from build123d import *

# Parameters (mm, degrees)
SKETCH1_W           = 49
SKETCH1_H           = 49
SKETCH1_W_2         = 4
SKETCH1_H_2         = 5
SKETCH1_W_3         = 3
BOSS_EXTRUDE1_DEPTH = 3


with BuildPart() as part:
    # Sketch1 → Boss-Extrude1 (new body)
    with BuildSketch(Plane(origin=(0, 0, 0), x_dir=(1, 0, 0), z_dir=(0, 1, 0))):
        Rectangle(SKETCH1_W, SKETCH1_H)
        with Locations((26.5, 0)):
            Rectangle(SKETCH1_W_2, SKETCH1_H_2)
        Polygon((-27.5, 27.5), (-27.5, 24.5), (-27.5, -24.5), (-27.5, -27.5), (-30.5, -27.5), (-30.5, 27.5), align=None)
        with Locations((-26, 0)):
            Rectangle(SKETCH1_W_3, SKETCH1_H)
    extrude(amount=BOSS_EXTRUDE1_DEPTH)


solid = part.part
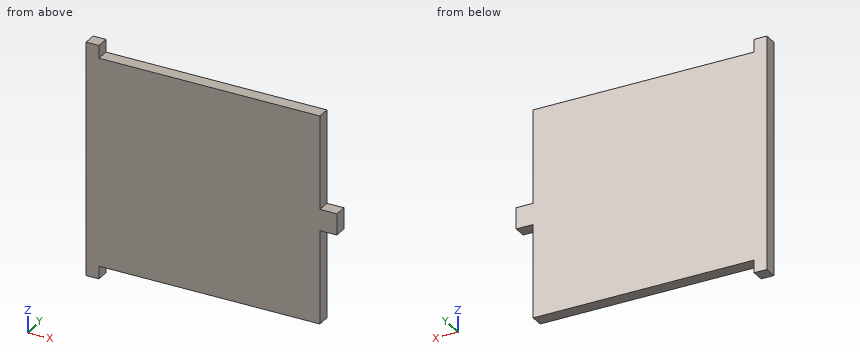
Design review of the part built by this model. Coordinates are the model's own, in mm. Round coordinates to 2 decimals unless told otherwise and drop trailing zeros. Write each loop counter-clockwise with the first axis right and the second up, starting at its lowest first coordinate (ties: lowest second). Pieces come first, ordered by that corner, then holes.
Item 1: Consider section C-C on x = -4. Give the boundary of the cut face in (y, z).
Item 2: Consider section A-A on y = 2.05. Give the boundary of the cut face in (x, z).
Item 3: For pin 1 Ø0.9 at (y, z) = (2, 25.5) entering from +X; pin 2 Ø0.9 at (x, y) = (26.5, 2) entering from +Z; pin 3 Ø0.9 at (x, y) = (25.5, 1.5) entering from -Z, all flat-tipped, find the tip position at first contact; note any pin that passes through.
Item 4: Wall thickness on L1, parallel to Z at x = -11.5, y = 1.7; L2, parallel to X at y = 0.9, z = -9.5: over which ranges is each line inside the solid? List them lowest first.
Item 5: Consider section B-B on z = 19.5. Give the boundary of the cut face in (x, y), and give its area (3 significant figures).
Check values:
1. outline: (0, -24.5) - (3, -24.5) - (3, 24.5) - (0, 24.5) - close
2. outline: (-30.5, -27.5) - (-27.5, -27.5) - (-27.5, -24.5) - (24.5, -24.5) - (24.5, -2.5) - (28.5, -2.5) - (28.5, 2.5) - (24.5, 2.5) - (24.5, 24.5) - (-27.5, 24.5) - (-27.5, 27.5) - (-30.5, 27.5) - close
3. pin 1: stops at x = -27.5
3. pin 2: stops at z = 2.5
3. pin 3: stops at z = -2.5
4. L1: z = -24.5 to 24.5
4. L2: x = -30.5 to 24.5
5. outline: (-30.5, 0) - (24.5, 0) - (24.5, 3) - (-30.5, 3) - close
5. area: 165 mm2
